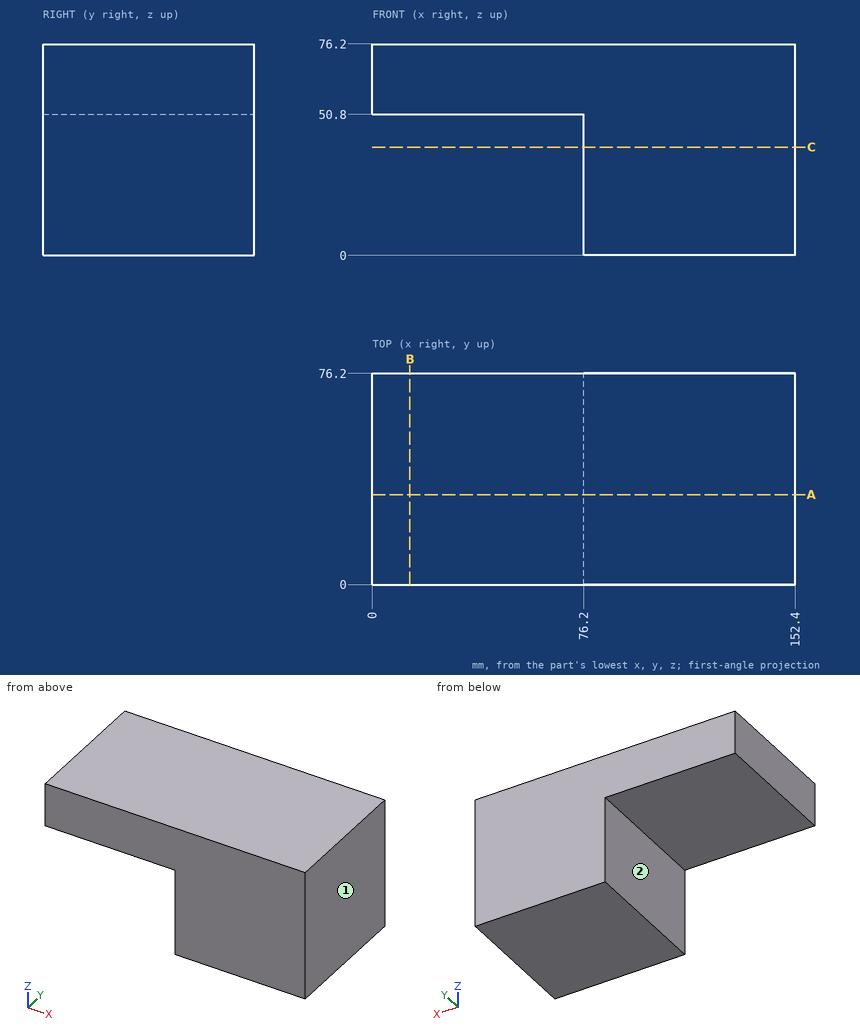
Drawing for the job (mm, zero at the part's lowest x, y, z). A direction names the side the tool comes from. Coordinates: 2 decimals unless noted, no trailing zeros. Order: outer loops, then holes, each group sorted by start corner. A loop starts at its lowest first (then second) coordinate and runs counter-clockwise, first axis right, second up. Notation, with made-up numbers: (80.25, 42) - (128.25, 42) arc R19 ccw to (128.25, 76) - close; hole circle Ø4 at (69, 49.5). An arc over 180 degrees is marked (long way). Use a Markdown table: item, result. Add a question column.
(1) Saw through at B-B (x = 13.5). Give the cut face in (y, z).
(2) Which spindle directions (+Z, -Z, +X, -X, +Y, -Y) get a long thin tool onto all of the face, cutting with end or side? Do the marked faces 1 and 2. Say none if no direction does.
(3) Flat gauge pins, fed straight in: pin 1 (15 mm diameter, centred on y = 48, z = 24.5, fed in from -X); pin 2 (4 mm diameter, centred on x = 57.5, y = 18, fed in from -Z). Where does each tip first touch, or does it go through?
(4) Saw through at A-A (y = 32.5). Give the cut face in (x, z).
(5) Drill centre lines: line 1 along X through (y, z) = (29, 12); line 2 along Z through (x, y) = (62, 66.5). Where is each one in solid material? Low to high. Write a range as [from, to].
(6) Saw through at C-C (z = 39). Give the cut face in (x, y), then the cut area to 3 significant figures.
Solved:
| question | item | result |
|---|---|---|
| 1 | outline | (0, 50.8) - (76.2, 50.8) - (76.2, 76.2) - (0, 76.2) - close |
| 2 | face 1 | +Z, -Z, +X, +Y, -Y |
| 2 | face 2 | -Z, -X, +Y, -Y |
| 3 | pin 1 | stops at x = 76.2 |
| 3 | pin 2 | stops at z = 50.8 |
| 4 | outline | (0, 50.8) - (76.2, 50.8) - (76.2, 0) - (152.4, 0) - (152.4, 76.2) - (0, 76.2) - close |
| 5 | line 1 | x = [76.2, 152.4] |
| 5 | line 2 | z = [50.8, 76.2] |
| 6 | outline | (76.2, 0) - (152.4, 0) - (152.4, 76.2) - (76.2, 76.2) - close |
| 6 | area | 5,810 mm² |
